```python
from build123d import *

# Parameters (mm, degrees)
BOSS_EXTRUDE1_DEPTH = 3
FILLET1_R           = 10
FILLET2_R           = 15
SKETCH2_R           = 2.5
CUT_EXTRUDE1_DEPTH  = 135.662541191


with BuildPart() as part:
    # Sketch1 → Boss-Extrude1 (new body)
    with BuildSketch(Plane(origin=(0, 0, 0), x_dir=(1, 0, 0), z_dir=(0, 1, 0))):
        Polygon((0, 115), (-30, 115), (-30, 30), (-70, 30), (-70, 0), (0, 0), align=None)
    extrude(amount=BOSS_EXTRUDE1_DEPTH)

    # Fillet1
    fillet1_edges = [part.edges().sort_by_distance(p)[0] for p in [
        (0, 1.5, -115),
        (-30, 1.5, -115),
        (-70, 1.5, -30),
        (-70, 1.5, 0),
    ]]
    fillet(fillet1_edges, radius=FILLET1_R)

    # Fillet2
    fillet2_edges = [part.edges().sort_by_distance(p)[0] for p in [
        (0, 1.5, 0),
    ]]
    fillet(fillet2_edges, radius=FILLET2_R)

    # Sketch2 → Cut-Extrude1 (cut, through all)
    with BuildSketch(Plane(origin=(0, 3, 0), x_dir=(1, 0, 0), z_dir=(0, 1, 0))):
        with Locations(Location((-60, 15, 0), (0, 0, 270))):
            Circle(SKETCH2_R)
        with Locations(Location((-15, 105, 0), (0, 0, 270))):
            Circle(SKETCH2_R)
    extrude(amount=-CUT_EXTRUDE1_DEPTH, mode=Mode.SUBTRACT)


solid = part.part
```
Can you work these out from the model? Positions are in its coordinate system, mm. A direction names the side the tool comes from. Round coordinates to 2 decimals unless told otherwise and drop trailing zeros. Loops run counter-clockwise (first coordinate to the right, second up) from the corner with the lowest first, then second, coordinate; pieces in that order, holes last. Notation, with made-up numbers: (-23.75, 24.25) -> (18.25, 24.25) arc R25 cw to (18.25, 56.25) -> close; hole circle Ø8 at (47, 32). An arc over 180 degrees is marked (long way). One line per item, written item: value. Start each with the question number.
1. For pin 1 (1.5 mm diameter, centred on x = -42.5, y = 2, fed in from -Z), with a flat end and sliding along its axis, tell me the tip position at first contact or that it passes through.
2. If I drill on probe 1 along X at (y, z) = (1.35, -81); probe 2 along Z at (x, y) = (-23, 1.9), over which ranges is the centre line in solid material (lowest first)?
3. If we section it at B-B, the plane z = -51: Write out the boundary of the cut face in (x, y), then the cut area to 3 significant figures.
4. If we section it at A-A, the plane y = 2.4: Write out the boundary of the cut face in (x, z).
5. For faces 4 (the flat face through (-70, 1, -15)), 5 (the flat face through (-30, 1, -68)), which set-ups out of +Z, -Z, +X, -X, +Y, -Y let a thin tool reach every point of the face, with its end or its side?
6. If we section it at C-C, the plane x = -36: Write out the boundary of the cut face in (y, z).
7. If we mould it in two halves opening along Z, with no side actions, what happens to faces 1 (the flat face through (0, 1, -59)), 2 (the cylindrical face through (-58.31, 1.52, -16.84)), 3 (the flat face through (-15, 1, -115))? For each: pulls with the +Z half, pulls with the -Z half, needs draft (parallel to the pull), parting line crosses it, or undercut.
Calculated:
1. pin 1: stops at z = -30
2. probe 1: x = -30 to 0
2. probe 2: z = -114.54 to 0
3. outline: (-30, 0) -> (0, 0) -> (0, 3) -> (-30, 3) -> close
3. area: 90.0 mm²
4. outline: (-70, -20) arc R10 ccw to (-60, -30) -> (-30, -30) -> (-30, -105) arc R10 ccw to (-20, -115) -> (-10, -115) arc R10 ccw to (0, -105) -> (0, -15) arc R15 ccw to (-15, 0) -> (-60, 0) arc R10 ccw to (-70, -10) -> close; hole circle Ø5 at (-60, -15); hole circle Ø5 at (-15, -105)
5. face 4: +Z, -Z, -X, +Y, -Y
5. face 5: -Z, -X, +Y, -Y
6. outline: (0, -30) -> (3, -30) -> (3, 0) -> (0, 0) -> close
7. face 1: needs draft
7. face 2: undercut
7. face 3: pulls with the -Z half
